from build123d import *

# Parameters (mm, degrees)
SKETCH1_R           = 4.8895
SKETCH1_R_2         = 1.3335
SKETCH1_R_3         = 1.651
SKETCH1_W           = 3.175
SKETCH1_H           = 25.4
BOSS_EXTRUDE2_DEPTH = 3.175
FILLET1_R           = 3.175


with BuildPart() as part:
    # Sketch1 → Boss-Extrude2 (new body)
    with BuildSketch(Plane.XY):
        Polygon((0, 3.175), (3.175, 3.175), (3.175, 0), (9.525, 0), (9.525, 3.175), (15.875, 3.175), (15.875, 0), (22.225, 0), (22.225, 3.175), (28.575, 3.175), (28.575, 0), (34.925, 0), (34.925, 3.175), (41.275, 3.175), (41.275, 0), (47.625, 0), (47.625, 3.175), (53.975, 3.175), (53.975, 0), (60.325, 0), (60.325, 3.175), (66.675, 3.175), (66.675, 0), (73.025, 0), (73.025, 3.175), (79.375, 3.175), (79.375, 0), (85.725, 0), (85.725, 3.175), (88.9, 3.175), (94.2848, 3.175), (94.2848, -34.925), (167.535593046, -34.925), (167.535593046, 3.175), (170.4848, 3.175), (170.4848, 53.975), (167.3098, 53.975), (167.3098, 73.025), (170.4848, 73.025), (170.4848, 98.425), (167.3098, 98.425), (167.3098, 123.825), (170.4848, 123.825), (170.4848, 149.225), (167.3098, 149.225), (167.3098, 174.625), (170.4848, 174.625), (170.4848, 200.025), (167.3098, 200.025), (167.3098, 225.425), (170.4848, 225.425), (170.4848, 238.125), (88.9, 238.125), (88.9, 243.205), (85.725, 243.205), (85.725, 255.905), (88.9, 255.905), (88.9, 268.605), (85.725, 268.605), (85.725, 281.305), (88.9, 281.305), (88.9, 294.005), (85.725, 294.005), (85.725, 306.705), (88.9, 306.705), (88.9, 311.785), (82.390448212, 318.294551788), (84.635512242, 320.539615818), (80.145384182, 325.029743879), (77.900320151, 322.784679849), (73.410192091, 327.274807909), (75.655256121, 329.519871939), (71.165128061, 334.01), (68.92006403, 331.76493597), (64.42993597, 336.25506403), (66.675, 338.500128061), (62.184871939, 342.990256121), (59.939807909, 340.745192091), (55.449679849, 345.235320151), (57.694743879, 347.480384182), (53.204615818, 351.970512242), (50.959551788, 349.725448212), (44.45, 356.235), (38.1, 356.235), (38.1, 359.41), (31.75, 359.41), (31.75, 356.235), (25.4, 356.235), (25.4, 359.41), (19.05, 359.41), (19.05, 356.235), (12.7, 356.235), (12.7, 359.41), (6.35, 359.41), (6.35, 356.235), (0, 356.235), (0, 257.175), (3.175, 257.175), (3.175, 231.775), (0, 231.775), (0, 206.375), (3.175, 206.375), (3.175, 180.975), (0, 180.975), (0, 155.575), (3.175, 155.575), (3.175, 130.175), (0, 130.175), (0, 104.775), (3.175, 104.775), (3.175, 79.375), (0, 79.375), (0, 53.975), (3.175, 53.975), (3.175, 42.175), (0, 42.175), (0, 28.575), align=None)
        with Locations((88.9, 232.41)):
            Circle(SKETCH1_R, mode=Mode.SUBTRACT)
        with Locations((59.3598, 191.77)):
            Circle(SKETCH1_R_2, mode=Mode.SUBTRACT)
        with Locations((59.3598, 71.12)):
            Circle(SKETCH1_R_2, mode=Mode.SUBTRACT)
        with Locations((160.9598, 71.12)):
            Circle(SKETCH1_R_2, mode=Mode.SUBTRACT)
        with Locations((160.9598, 191.77)):
            Circle(SKETCH1_R_2, mode=Mode.SUBTRACT)
        with Locations((45.225, 66.574999946)):
            Circle(SKETCH1_R_3, mode=Mode.SUBTRACT)
        with Locations((45.225, 117.374999946)):
            Circle(SKETCH1_R_3, mode=Mode.SUBTRACT)
        with Locations((45.225, 168.174999946)):
            Circle(SKETCH1_R_3, mode=Mode.SUBTRACT)
        with Locations((157.7848, 5.969)):
            Circle(SKETCH1_R_3, mode=Mode.SUBTRACT)
        with Locations((87.3125, 123.825)):
            Rectangle(SKETCH1_W, SKETCH1_H, mode=Mode.SUBTRACT)
        Polygon((99.742302456, 1.4986), (102.917302456, -4.000661314), (100.321651116, -5.499261314), (97.146651116, 0), align=None, mode=Mode.SUBTRACT)
        with Locations((87.3125, 73.025)):
            Rectangle(SKETCH1_W, SKETCH1_H, mode=Mode.SUBTRACT)
        with Locations((87.3125, 22.225)):
            Rectangle(SKETCH1_W, SKETCH1_H, mode=Mode.SUBTRACT)
        Polygon((106.092302456, -9.499922628), (103.496651116, -10.998522628), (106.671651116, -16.497783942), (109.267302456, -14.999183942), align=None, mode=Mode.SUBTRACT)
        Polygon((113.854167186, -19.62934866), (112.355567186, -22.225), (117.8548285, -25.4), (119.3534285, -22.80434866), align=None, mode=Mode.SUBTRACT)
        Polygon((124.852689814, -25.97934866), (123.354089814, -28.575), (128.853351128, -31.75), (130.351951128, -29.15434866), align=None, mode=Mode.SUBTRACT)
    extrude(amount=BOSS_EXTRUDE2_DEPTH)

    # Fillet1
    fillet1_edges = [part.edges().sort_by_distance(p)[0] for p in [
        (88.9, 238.125, 1.5875),
        (167.535593046, -34.925, 1.5875),
        (94.2848, -34.925, 1.5875),
    ]]
    fillet(fillet1_edges, radius=FILLET1_R)


solid = part.part
Input: part model. Units: mm. Frame: model coordinates. Coordinates: 2 decimals unless noted, no trailing zeros. Loops run counter-clockwise (first coordinate to the right, second up) from the corner with the lowest first, then second, coordinate; pieces in that order, holes last.
(1) Section A-A on y = 249. Return the cut outline in (x, z) (3 decimals), then the cut area to 3 significant figures.
(2) Pull-direction query (Y, two-part tool) for faces 1 (the face through (47.75, 352.935, 1.565)), 2 (the face through (84, 165, 0)), 3 (the face through (85.691, 314.994, 1.565)), 4 (the face through (91.53, 236.53, 1.57)); classes: released by +Y, released by -Y, zero draft, split by the parting line, or undercut.
(3) Section B-B on z = 1.25. Count the separate pieces of the cut face and the enclosed holes in it, then the cut area to 3 significant figures.
(4) First-contact query: pin 1 Ø0.6 at (y, z) = (242.5, 1.5) entering from +X; pin 2 Ø1.6 at (x, z) = (88, 1) entering from -Y (3 decimals); pin 3 Ø1 at (y, z) = (357, 1.5) entering from -X. Flat tips, straight axial feed; report the tip coordinate or a pass-through.
(5) Material intervals for probe 1 along X at (y, z) = (191.77, 1.2) (3 decimals); probe 2 along X at (y, z) = (122.5, 2.6) (3 decimals); probe 3 along Y at (x, z) = (119, 0.6) (1 decimal), sorted ascending.
(6) Section C-C on y = 46. Return the cut outline in (x, z) (3 decimals), then the cut area to 3 significant figures.
Data:
1. outline: (3.175, 0) - (85.725, 0) - (85.725, 3.175) - (3.175, 3.175) - close
1. area: 262 mm2
2. face 1: released by +Y
2. face 2: zero draft
2. face 3: undercut
2. face 4: undercut
3. separate pieces: 1
3. enclosed holes: 16
3. area: 51,400 mm2
4. pin 1: stops at x = 88.9
4. pin 2: stops at y = 3.175
4. pin 3: stops at x = 6.35
5. probe 1: x = 3.175 to 58.026, 60.693 to 159.626, 162.293 to 170.485
5. probe 2: x = 0 to 85.725, 88.9 to 167.31
5. probe 3: y = -34.9 to -23.4, -22.6 to 238.1
6. outline: (3.175, 0) - (170.485, 0) - (170.485, 3.175) - (3.175, 3.175) - close
6. area: 531 mm2
